Source: CAD feature listing. Evaluate the final solid. Frame: model axes, mm. A direction names the side the tool comes from. Coordinates: 2 decimals unless noted, no trailing zeros. Order: outer loops, then holes, each group sorted by start corner. A loop starts at its lowest first (then second) coordinate and runs counter-clockwise, first axis right, second up.
Item 1: Contact query for flat-ended pins moving along their axis: P1, Ø2, axis at x = -5, z = 4.5, coming from the -Y side; P2, Ø4, axis at x = -7.5, y = -10.5, coming from the -Z side; P3, Ø2, axis at y = 13.5, z = 2.5, coming from the +X side; P4, Ø12, axis at x = -13.5, y = 6, coming from the -Z side. Output: stop coordinate, or through.
Item 2: Ray query, line 1 (Y direction, x = 0, z = 5.5); line 2 (Y direction, x = -13, z = 7.5); line 3 (X direction, y = -5.5, z = 6). Return the intervals inside material, ascending.
Item 3: Section C-C on z = 1.25. Return the cut outline in (x, y), then the cut area to 3 significant figures.
Item 4: Section D-D on x = 19.5. Return the cut outline in (y, z).
Item 5: Section A-A on x = 0. Return the cut outline in (y, z).
Item 6: Reachability of faces 1 (the flat face through (7, -20, 2)), 2 (the cylindrical face through (-14.985, 0.66, 5.07)) from +Z, -Z, +X, -X, +Y, -Y: full face, straight path, thin tool, end or side. Return the list, or none.
from build123d import *

# Parameters (mm, degrees)
SKETCH1_R           = 21
SKETCH1_R_2         = 15
BOSS_EXTRUDE1_DEPTH = 10
SKETCH6_R           = 22.5
BOSS_EXTRUDE2_DEPTH = 2
SKETCH7_R           = 15
CUT_EXTRUDE1_DEPTH  = 34.35416016


with BuildPart() as part:
    # Sketch1 → Boss-Extrude1 (new body)
    with BuildSketch(Plane.XY):
        Circle(SKETCH1_R)
        Circle(SKETCH1_R_2, mode=Mode.SUBTRACT)
    extrude(amount=BOSS_EXTRUDE1_DEPTH)

    # Sketch6 → Boss-Extrude2 (add)
    with BuildSketch(Plane(origin=(0, 0, 0), x_dir=(-1, 0, 0), z_dir=(0, 0, -1))):
        Circle(SKETCH6_R)
    extrude(amount=-BOSS_EXTRUDE2_DEPTH)

    # Sketch7 → Cut-Extrude1 (cut, through all)
    with BuildSketch(Plane.XY.offset(10)):
        Circle(SKETCH7_R)
    extrude(amount=-CUT_EXTRUDE1_DEPTH, mode=Mode.SUBTRACT)


solid = part.part
Answer list:
1. P1: stops at y = -20.62
1. P2: passes through
1. P3: stops at x = 18.62
1. P4: stops at z = 0
2. line 1: y = -21 to -15, 15 to 21
2. line 2: y = -16.49 to -7.48, 7.48 to 16.49
2. line 3: x = -20.27 to -13.96, 13.96 to 20.27
3. outline: circle Ø45 at (0, 0); hole circle Ø30 at (0, 0)
3. area: 884 mm2
4. outline: (-11.22, 0) - (11.22, 0) - (11.22, 2) - (7.79, 2) - (7.79, 10) - (-7.79, 10) - (-7.79, 2) - (-11.22, 2) - close
5. outline: (-22.5, 0) - (-15, 0) - (-15, 10) - (-21, 10) - (-21, 2) - (-22.5, 2) - close; (15, 0) - (22.5, 0) - (22.5, 2) - (21, 2) - (21, 10) - (15, 10) - close
6. face 1: +Z
6. face 2: +Z, -Z
